Verification items for the finished model (mm, model axes). A direction names the side the tool comes from. Give positions to 0.01 mm unless a question says otherwise; leave off trailing zeros. Write each loop counter-clockwise with the first axis right and the second up, starting at its lowest first coordinate (ties: lowest second). Pieces come first, ordered by that corner, then holes. Notation, with made-up numbers: M 24.25,-31 L 81.25,-31 A22 cw 81.25,6 Z; hole C 6.5,21.25 d7. An arc over 180 degrees is marked long. Answer as a JSON object with one key per item and string values.
```python
from build123d import *

# Parameters (mm, degrees)
SKETCH1_R           = 28.70835
BOSS_EXTRUDE1_DEPTH = 15.50924
FILLET1_R           = 7.75462
SKETCH2_R           = 19.05
CUT_EXTRUDE2_DEPTH  = 6.604
CUT_EXTRUDE3_START  = -6.604
SKETCH3_R           = 19.05
CUT_EXTRUDE3_DEPTH  = 6.604
SKETCH4_R           = 5.588
SKETCH4_R_2         = 4.572
BOSS_EXTRUDE2_DEPTH = 2.032
CUT_EXTRUDE4_START  = -11.43
SKETCH5_R           = 4.572
CUT_EXTRUDE4_DEPTH  = 11.43
SKETCH6_R           = 1.524
CUT_EXTRUDE5_DEPTH  = 11.43
CIRPATTERN1_COUNT   = 3
SKETCH10_R          = 0.762
CUT_EXTRUDE8_DEPTH  = 11.43
CIRPATTERN3_COUNT   = 3
FILLET2_R           = 0.254
FILLET3_R           = 0.254


with BuildPart() as part:
    # Sketch1 → Boss-Extrude1 (new body)
    with BuildSketch(Plane.XY):
        Circle(SKETCH1_R)
    extrude(amount=BOSS_EXTRUDE1_DEPTH)

    # Fillet1
    fillet1_edges = [part.edges().sort_by_distance(p)[0] for p in [
        (-28.70835, 0, 0),
        (-28.70835, 0, 15.50924),
    ]]
    fillet(fillet1_edges, radius=FILLET1_R - 0.0001)  # a hair under: the kernel refuses the full size

    # Sketch2 → Cut-Extrude2 (cut)
    with BuildSketch(Plane.XY.offset(15.50924)):
        Circle(SKETCH2_R)
    extrude(amount=-CUT_EXTRUDE2_DEPTH, mode=Mode.SUBTRACT)

    # Sketch3 → Cut-Extrude3 (cut)
    with BuildSketch(Plane(origin=(0, 0, 0), x_dir=(-1, 0, 0), z_dir=(0, 0, -1)).offset(CUT_EXTRUDE3_START)):
        with Locations(Location((0, 0, 0), (0, 0, 180))):
            Circle(SKETCH3_R)
    extrude(amount=CUT_EXTRUDE3_DEPTH, mode=Mode.SUBTRACT)

    # Sketch4 → Boss-Extrude2 (add)
    with BuildSketch(Plane.XY.offset(8.90524)):
        Circle(SKETCH4_R)
        Circle(SKETCH4_R_2, mode=Mode.SUBTRACT)
    boss_extrude2 = extrude(amount=BOSS_EXTRUDE2_DEPTH)

    # Sketch5 → Cut-Extrude4 (cut)
    with BuildSketch(Plane.XY.offset(8.90524).offset(CUT_EXTRUDE4_START)):
        with Locations(Location((0, 0, 0), (0, 0, 180))):
            Circle(SKETCH5_R)
    extrude(amount=CUT_EXTRUDE4_DEPTH, mode=Mode.SUBTRACT)

    # Mirror4: Boss-Extrude2 across plane
    add(boss_extrude2.mirror(Plane.XY.offset(7.75462)))

    # Sketch6 → Cut-Extrude5 (cut)
    with BuildSketch(Plane.XY.offset(8.90524)):
        with Locations((0, 9.906)):
            Circle(SKETCH6_R)
    cut_extrude5 = extrude(amount=-CUT_EXTRUDE5_DEPTH, mode=Mode.SUBTRACT)

    # CirPattern1: Cut-Extrude5 ×3 about axis
    cirpattern1_axis = Axis((0, 0, 0), (0, 0, 1))
    for i in range(1, CIRPATTERN1_COUNT):
        add(cut_extrude5.rotate(cirpattern1_axis, i * 360 / CIRPATTERN1_COUNT), mode=Mode.SUBTRACT)

    # Sketch10 → Cut-Extrude8 (cut)
    with BuildSketch(Plane.XY.offset(8.90524)):
        with Locations((0, -8.382)):
            Circle(SKETCH10_R)
    cut_extrude8 = extrude(amount=-CUT_EXTRUDE8_DEPTH, mode=Mode.SUBTRACT)

    # CirPattern3: Cut-Extrude8 ×3 about axis
    cirpattern3_axis = Axis((0, 0, 0), (0, 0, 1))
    for i in range(1, CIRPATTERN3_COUNT):
        add(cut_extrude8.rotate(cirpattern3_axis, i * 360 / CIRPATTERN3_COUNT), mode=Mode.SUBTRACT)

    # Fillet2
    fillet2_edges = [part.edges().sort_by_distance(p)[0] for p in [
        (-5.588, 0, 10.93724),
    ]]
    fillet(fillet2_edges, radius=FILLET2_R)

    # Fillet3
    fillet3_edges = [part.edges().sort_by_distance(p)[0] for p in [
        (-5.588, 0, 4.572),
    ]]
    fillet(fillet3_edges, radius=FILLET3_R)


solid = part.part
```
1) Section check D-D on z = 1.25. Record the boundary of the cut face in (x, y).
Completed:
{"outline": "C 0,0 d50.35; hole C 0,0 d38.1"}
2) Section check C-C on z = 13.75. Record the boundary of the cut face in (x, y).
Completed:
{"outline": "C 0,0 d51.74; hole C 0,0 d38.1"}
3) Access from +Z, -Z, +X, -X, +Y, -Y to the whole of each face (thin tool, end or side, straight path). Record for faces 3 (the face through (-5, 4, 6.604)), 4 (the face through (7.669, 4.834, 7.771)), 5 (the face through (-4.434, -3.4, 9.782)).
Completed:
{"face 3": "-Z", "face 4": "+Z, -Z", "face 5": "+Z"}
4) Thickness scan on L1, parallel to X at y = -1, z = 9.5; L2, parallel to Y at x = 0, z = 5.4; L3, parallel to Y at x = -1, z = 5.25. Record the ranges inside material, lowest first.
Completed:
{"L1": "x = -28.49 to -19.02, -5.5 to -4.46, 4.46 to 5.5, 19.02 to 28.49", "L2": "y = -28.34 to -19.05, -5.59 to -4.57, 4.57 to 5.59, 19.05 to 28.34", "L3": "y = -28.28 to -19.02, -5.5 to -4.46, 4.46 to 5.5, 19.02 to 28.28"}
5) Go/stop test with flat-tipped pins: pin 1 (8 mm diameter, centred on x = 0, y = 0, fed in from +Z); pin 2 (10.5 mm diameter, centred on x = 0, y = 0, fed in from -Z); pin 3 (4 mm diameter, centred on y = 13, z = 12.5, fed in from +X); pin 4 (6 mm diameter, centred on y = -11, z = 13.5, fed in from -X). Record where each tip stops, or that it passes through.
Completed:
{"pin 1": "passes through", "pin 2": "stops at z = 4.57", "pin 3": "stops at x = 25.45", "pin 4": "stops at x = -26.39"}
6) Release check for a two-part mould opening along Y. For faces 1 (the face through (5, -19, 15.509)), 2 (the face through (-0.099, -7.626, 7.771)) record: pulls with the +Y half, pulls with the -Y half, needs draft (parallel to the pull), parting line crosses it, or undercut.
Completed:
{"face 1": "needs draft", "face 2": "undercut"}
7) Section check B-B on x = 0. Count the separate pieces of the cut face and the enclosed holes in it, and give its area (3 significant figures).
Completed:
{"separate pieces": "4", "enclosed holes": "0", "area": "312 mm2"}
